Autodesk Inventor part; units mm, degrees
ref_plane "YZ Plane" through (0, 0, 0) normal (1, 0, 0) x (0, 1, 0)
ref_plane "XZ Plane" through (0, 0, 0) normal (0, 1, 0) x (-1, 0, 0)
ref_plane "XY Plane" through (0, 0, 0) normal (0, 0, 1) x (1, 0, 0)
sketch "Sketch1" plane through (0, 0, 0) normal (0, 0, 1) x (1, 0, 0)
  line L0 (-39, 50) -> (6, 50)
  line L1 (6, 50) -> (6, 44)
  line L2 (6, 44) -> (-39, 44)
  line L3 (-39, 44) -> (-39, 50)
  line L4 (0, 44) -> (6, 44)
  line L5 (6, 44) -> (6, 0)
  line L6 (6, 0) -> (0, 0)
  line L7 (0, 0) -> (0, 44)
  dimension "d1" = 6
  dimension "d2" = 45
  dimension "d3" = 6
  dimension "d17" = 50
extrude "Extrusion1" add sketch "Sketch1" along normal blind 3
fillet "Fillet1" radius 15 1 edges at (0, 44, 1.5)
sketch "Sketch2" plane through (0, 0, 3) normal (0, 0, 1) x (1, 0, 0)
  line L0 (6, 50) -> (-39, 50)
  line L1 (6, 0) -> (6, 50)
  point P0 (0, 0)
  point P1 (0, 44)
  dimension "d8" = 6
  dimension "d9" = 6
hole "Hole1" at (0, 44, 3) direction (0, 0, -1) diameter 5.5 end through all
equation "\"d3\" = d1"
properties part number "Selection_Selector 1" material "Nylon 6/6"
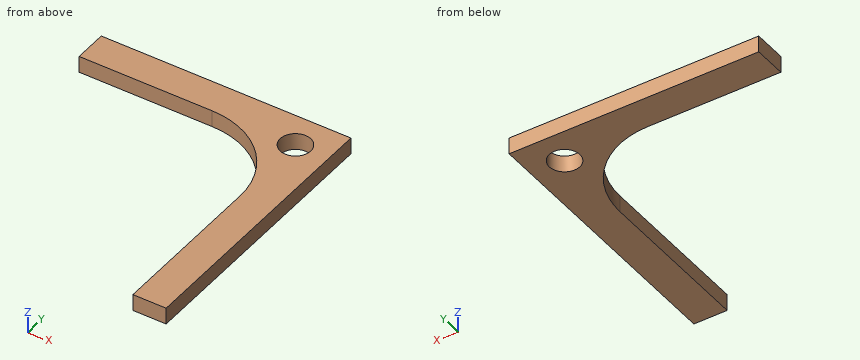
Check sheet for the modelled part. Datum: model origin and axes. Units: mm. Give positions to 0.01 mm unless a question says otherwise; leave off trailing zeros. Write each loop counter-clockwise with the first axis right and the second up, starting at its lowest first coordinate (ties: lowest second). Pieces come first, ordered by that corner, then holes. Notation, with made-up numbers: (25.25, 73.5) -> (63.25, 73.5) arc R9 cw to (63.25, 83.5) -> close; hole circle Ø1 at (8.5, 69.5). An arc over 180 degrees is marked (long way). Use CSV: the item, a comma, the result in double quotes. Start each with the question number.
Q1. Scan lines: line 1 along X through (y, z) = (17.5, 1.7); line 2 along Y through (x, z) = (-32, 2.6); line 3 along Y through (x, z) = (-5.5, 2.4). Record each from-to range of solid material in increasing order.
Q2. Cross-section at B-B on x = -28.5. Enter the section's corners in (y, z).
Q3. Cross-section at C-C on y = 38.5. Enter the section's corners in (x, z), and give its area (3 significant figures).
Q4. Cross-section at A-A on z = 2.2. Enter the section's corners in (x, y).
Q5. Depth check by flat-ended pin: P1, Ø1.5, axis at y = 25.5, z = 2.5, coming from the -X side; P2, Ø3.5, axis at x = 0, y = 44, coming from the +Z side. Enter the tip coordinate at first touch or a pass-through.
Working result:
1,line 1,"x = 0 to 6"
1,line 2,"y = 44 to 50"
1,line 3,"y = 40.61 to 50"
2,outline,"(44, 0) -> (50, 0) -> (50, 3) -> (44, 3) -> close"
3,outline,"(-3.39, 0) -> (6, 0) -> (6, 3) -> (-3.39, 3) -> close"
3,area,"28.2 mm^2"
4,outline,"(-39, 44) -> (-15, 44) arc R15 cw to (0, 29) -> (0, 0) -> (6, 0) -> (6, 50) -> (-39, 50) -> close; hole circle Ø5.5 at (0, 44)"
5,P1,"stops at x = 0"
5,P2,"passes through"
